Source: three-view drawing plus pictorial views. Frame: mm from the lowest corner of the part. A direction names the side the tool comes from. Round coordinates to 2 decimals unless told otherwise and drop trailing zeros. Order: outer loops, then holes, each group sorted by start corner. A loop starts at its lowest first (then second) coordinate and runs counter-clockwise, first axis right, second up. Notation, with made-up numbers: M 75,40.5 L 91,40.5 A33 cw 91,78.5 Z; hole C 36,45.5 d3. An arc over 180 degrees is marked long. Return JSON: item names as keys, results as strings. Group by question number.
Q1. Contact query for flat-ended pins moving along their axis: pin 1 (14 mm diameter, centred on x = 52, y = 10, fed in from +Z) (1 decimal); pin 2 (2 mm diameter, centred on x = 15.66, z = 59.79, fed in from -Y); pin 3 (4 mm diameter, centred on x = 76, z = 23, fed in from +Y); pin 4 (3 mm diameter, centred on x = 73.66, z = 10.795, fed in from -Y). Output: stop coordinate, or through.
Q2. Cut plane C-C on x = 73.66. Output: boundary loops of the cut face in (y, z) (1 decimal), and give its area (3 significant figures).
Q3. Access query for the marked faces 1, 2 and 3. Directions: +Z, -Z, +X, -X, +Y, -Y. A direction counts if a zero-diameter tool reaches every point of the face in a straight line with its end or side. Return the directions, or none.
Q4. Cut plane D-D on z = 62.5. Output: boundary loops of the cut face in (x, y).
Q5. Cut plane A-A on y = 30.48. Output: boundary loops of the cut face in (x, z) (1 decimal).
Q6. Ray query, probe 1 along Z at (x, y) = (73.66, 19.55) (1 decimal); probe 2 along Y at (x, z) = (7.62, 1.5) (1 decimal); probe 3 along Z at (x, y) = (73, 18) (1 decimal). Return the intervals inside material, ascending.
Q7. Cut plane B-B on x = 93.98. Output: boundary loops of the cut face in (y, z) (1 decimal).
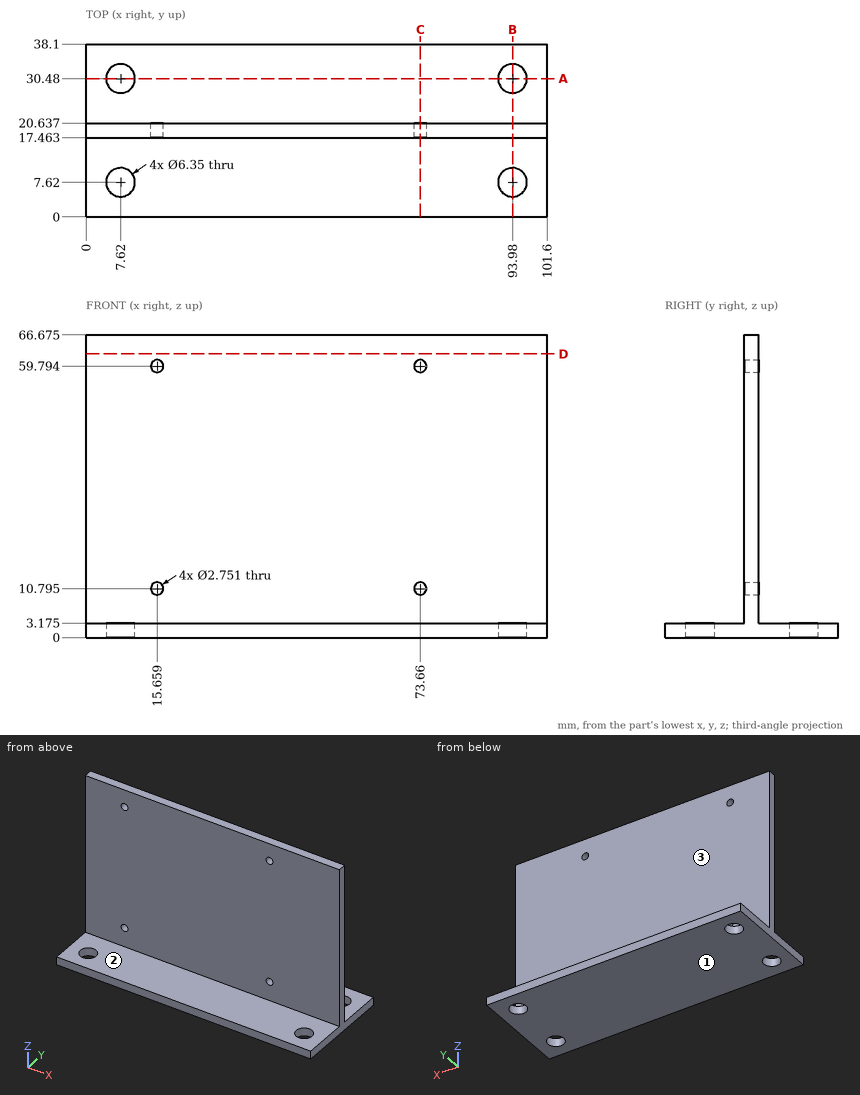
Result sheet:
{
 "1": {"pin 1": "stops at z = 3.2", "pin 2": "passes through", "pin 3": "stops at y = 20.64", "pin 4": "stops at y = 17.46"},
 "2": {"outline": "M 0,0 L 38.1,0 L 38.1,3.2 L 20.6,3.2 L 20.6,9.4 L 17.5,9.4 L 17.5,3.2 L 0,3.2 Z; M 17.5,12.2 L 20.6,12.2 L 20.6,58.4 L 17.5,58.4 Z; M 17.5,61.2 L 20.6,61.2 L 20.6,66.7 L 17.5,66.7 Z", "area": "305 mm²"},
 "3": {"face 1": "-Z, +X, -X, +Y, -Y", "face 2": "+Z, +X, -X, -Y", "face 3": "+Z, +X, -X, +Y"},
 "4": {"outline": "M 0,17.46 L 101.6,17.46 L 101.6,20.64 L 0,20.64 Z"},
 "5": {"outline": "M 0,0 L 4.4,0 L 4.4,3.2 L 0,3.2 Z; M 10.8,0 L 90.8,0 L 90.8,3.2 L 10.8,3.2 Z; M 97.2,0 L 101.6,0 L 101.6,3.2 L 97.2,3.2 Z"},
 "6": {"probe 1": "z = 0 to 9.4, 12.2 to 58.4, 61.2 to 66.7", "probe 2": "y = 0 to 4.4, 10.8 to 27.3, 33.7 to 38.1", "probe 3": "z = 0 to 9.6, 12 to 58.6, 61 to 66.7"},
 "7": {"outline": "M 0,0 L 4.4,0 L 4.4,3.2 L 0,3.2 Z; M 10.8,0 L 27.3,0 L 27.3,3.2 L 20.6,3.2 L 20.6,66.7 L 17.5,66.7 L 17.5,3.2 L 10.8,3.2 Z; M 33.7,0 L 38.1,0 L 38.1,3.2 L 33.7,3.2 Z"}
}
